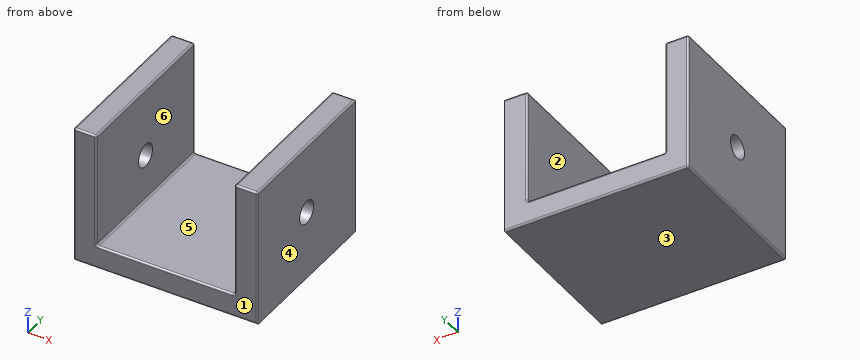
```python
from build123d import *

# Parameters (mm, degrees)
F1_DEPTH = 44.45
F3_D     = 6.35
F4_R     = 0.508


with BuildPart() as f1:
    # F0 (on Front) → F1 (new body)
    with BuildSketch(Plane.XZ):
        Polygon((19.05, 0), (0, 0), (-19.05, 0), (-19.05, 31.75), (-25.4, 31.75), (-25.4, -6.35), (25.4, -6.35), (25.4, 31.75), (19.05, 31.75), align=None)
    extrude(amount=F1_DEPTH)

    # F3 (through all)
    with Locations(Plane.YZ.offset(25.4)):
        with Locations((-22.225, 12.7)):
            Hole(F3_D / 2)

    # F4
    f4_edges = [f1.edges().sort_by_distance(p)[0] for p in [
        (-19.05, -22.225, 31.75),
        (19.05, -22.225, 31.75),
        (25.4, -22.225, 31.75),
        (22.225, -44.45, 31.75),
        (22.225, 0, 31.75),
        (25.4, -44.45, 12.7),
        (19.05, -44.45, 15.875),
        (0, -44.45, 0),
        (19.05, -22.225, 0),
        (-19.05, -22.225, 0),
        (0, 0, 0),
        (-19.05, -44.45, 15.875),
        (-19.05, 0, 15.875),
        (-25.4, -22.225, 31.75),
        (-22.225, 0, 31.75),
        (-22.225, -44.45, 31.75),
        (-25.4, -44.45, 12.7),
        (0, -44.45, -6.35),
        (0, 0, -6.35),
        (-25.4, 0, 12.7),
        (19.05, 0, 15.875),
        (-25.4, -22.225, -6.35),
    ]]
    fillet(f4_edges, radius=F4_R)


solid = f1.part
```
The listing builds one solid part. Answer for the finished solid, in the listing's coordinates (mm). Face numbers are marked on the shaded views. A direction names the side the tool comes from. Give positions to 0.01 mm unless a question says otherwise; leave off trailing zeros. Order: outer loops, then holes, each group sorted by start corner. A loop starts at its lowest first (then second) coordinate and runs counter-clockwise, first axis right, second up. Notation, with made-up numbers: M 55,81.25 L 73,81.25 A19 ccw 73,107.25 Z; hole C 84,71 d3. An arc over 180 degrees is marked long. Put each result on its own line as item: value. Start each with the question number.
Item 1: The part is cut by section D-D, the plane x = 4.5. Determine the outline of the cut face in (y, z).
Item 2: Which of the six approach directions +Z, -Z, +X, -X, +Y, -Y give full straight-line access (tool end or side, diameter ignored) to the marked faces 1 and 2?
Item 3: The part is cut by section A-A, the plane z = 12.7. Determine the outline of the cut face in (x, y).
Item 4: Flat-ended cylindrical pins translate along their axes: P1, Ø4, axis at x = 17, z = 11.5, coming from the +Y side; P2, Ø1, axis at x = -4, y = -7.5, coming from the +Z side. Find the tip coordinate at first contact, or state that the pin passes through.
Item 5: For a pull along X with two mould halves and no side action, classify the marked faces 3, 4, 5 and 6 as +X half, -X half, draft (parallel to the pull), parting line (faces both ways), or undercut.
Item 6: The part is cut by section B-B, the plane z = 6.5. Determine the outline of the cut face in (x, y).
Item 7: The part is cut by section C-C, the plane y = -32. Determine the outline of the cut face in (x, z).
Item 8: Find the intervals of material crossed by line 1 along X through (y, z) = (-12, 22); line 2 along Z through (x, y) = (5, -17.5); line 3 along Y through (x, z) = (22, 12), in increasing order.
Answer key:
1. outline: M -44.45,-5.84 A0.51 ccw -43.94,-6.35 L -0.51,-6.35 A0.51 ccw 0,-5.84 L 0,-0.51 A0.51 ccw -0.51,0 L -43.94,0 A0.51 ccw -44.45,-0.51 Z
2. face 1: +Z, -Z, +X, -X, -Y
2. face 2: +Z, +Y, -Y
3. outline: M -25.4,-43.94 A0.51 ccw -24.89,-44.45 L -19.56,-44.45 A0.51 ccw -19.05,-43.94 L -19.05,-25.4 L -25.4,-25.4 Z; M -25.4,-19.05 L -19.05,-19.05 L -19.05,-0.51 A0.51 ccw -19.56,0 L -24.89,0 A0.51 ccw -25.4,-0.51 Z; M 19.05,-43.94 A0.51 ccw 19.56,-44.45 L 24.89,-44.45 A0.51 ccw 25.4,-43.94 L 25.4,-25.4 L 19.05,-25.4 Z; M 19.05,-19.05 L 25.4,-19.05 L 25.4,0 L 19.56,0 A0.51 ccw 19.05,-0.51 Z
4. P1: passes through
4. P2: stops at z = 0
5. face 3: draft
5. face 4: +X half
5. face 5: undercut
5. face 6: undercut
6. outline: M -25.4,-43.94 A0.51 ccw -24.89,-44.45 L -19.56,-44.45 A0.51 ccw -19.05,-43.94 L -19.05,-0.51 A0.51 ccw -19.56,0 L -24.89,0 A0.51 ccw -25.4,-0.51 Z; M 19.05,-43.94 A0.51 ccw 19.56,-44.45 L 24.89,-44.45 A0.51 ccw 25.4,-43.94 L 25.4,0 L 19.56,0 A0.51 ccw 19.05,-0.51 Z
7. outline: M -25.4,-5.84 A0.51 ccw -24.89,-6.35 L 25.4,-6.35 L 25.4,31.24 A0.51 ccw 24.89,31.75 L 19.56,31.75 A0.51 ccw 19.05,31.24 L 19.05,0.51 A0.51 cw 18.54,0 L -18.54,0 A0.51 cw -19.05,0.51 L -19.05,31.24 A0.51 ccw -19.56,31.75 L -24.89,31.75 A0.51 ccw -25.4,31.24 Z
8. line 1: x = -25.4 to -19.05, 19.05 to 25.4
8. line 2: z = -6.35 to 0
8. line 3: y = -44.45 to -25.32, -19.13 to 0
